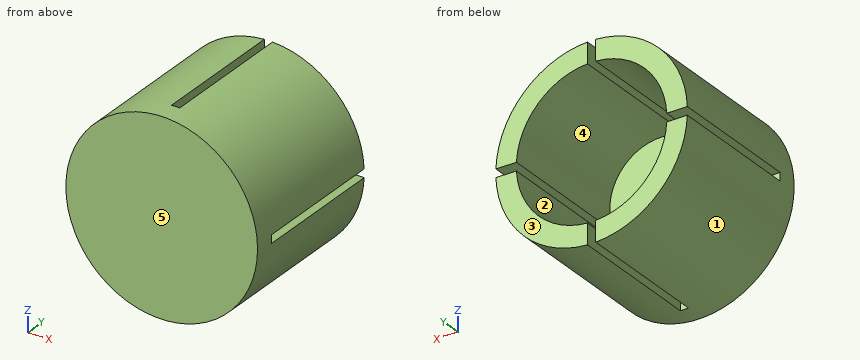
```python
from build123d import *

# Parameters (mm, degrees)
CUT_EXTRUDE1_DEPTH = 20


with BuildPart() as part:
    # Sketch2 → Revolve1 (revolve)
    with BuildSketch(Plane.XY, mode=Mode.PRIVATE) as revolve1_sk:
        Polygon((0, 0), (14, 0), (14, 23), (11, 23), (11, 3), (7.5, 3), (7.5, 8), (0, 8), align=None)
    revolve(revolve1_sk.sketch.rotate(Axis((0, 8, 0), (0, -1, 0)), 180), axis=Axis((0, 8, 0), (0, -1, 0)))

    # Sketch3 → Cut-Extrude1 (cut)
    with BuildSketch(Plane(origin=(0, 23, 0), x_dir=(1, 0, 0), z_dir=(0, 1, 0))):
        with BuildLine():
            ThreePointArc((-0.6, -13.987136948), (-0.300068933, -13.996783868), (0, -14))
            ThreePointArc((0, -14), (0.300068933, -13.996783868), (0.6, -13.987136948))
            Line((0.6, -13.987136948), (0.6, -10.983624174))
            ThreePointArc((0.6, -10.983624174), (0, -11), (-0.6, -10.983624174))
            Line((-0.6, -10.983624174), (-0.6, -13.987136948))
        make_face()
        with BuildLine():
            Line((-0.6, 13.987136948), (-0.6, 10.983624174))
            ThreePointArc((-0.6, 10.983624174), (0, 11), (0.6, 10.983624174))
            Line((0.6, 10.983624174), (0.6, 13.987136948))
            ThreePointArc((0.6, 13.987136948), (0.300068933, 13.996783868), (0, 14))
            ThreePointArc((0, 14), (-0.300068933, 13.996783868), (-0.6, 13.987136948))
        make_face()
        with BuildLine():
            ThreePointArc((-14, 5.1e-08), (-13.996783868, -0.300068907), (-13.987136948, -0.6))
            Line((-13.987136948, -0.6), (-10.983624174, -0.6))
            ThreePointArc((-10.983624174, -0.6), (-11, 0), (-10.983624174, 0.6))
            Line((-10.983624174, 0.6), (-13.987136948, 0.6))
            ThreePointArc((-13.987136948, 0.6), (-13.996783867, 0.300068958), (-14, 5.1e-08))
        make_face()
        with BuildLine():
            Line((10.983624174, -0.6), (13.987136948, -0.6))
            ThreePointArc((13.987136948, -0.6), (13.996783868, -0.300068933), (14, 0))
            ThreePointArc((14, 0), (13.996783868, 0.300068933), (13.987136948, 0.6))
            Line((13.987136948, 0.6), (10.983624174, 0.6))
            ThreePointArc((10.983624174, 0.6), (10.995905281, 0.300111716), (11, 0))
            ThreePointArc((11, 0), (10.995905281, -0.300111716), (10.983624174, -0.6))
        make_face()
    extrude(amount=-CUT_EXTRUDE1_DEPTH, mode=Mode.SUBTRACT)


solid = part.part
```
Work out the finished part from the listing and answer in its coordinate system (mm). Face numbers are marked on the shaded views. A direction names the side the tool comes from. Coordinates: 2 decimals unless noted, no trailing zeros. Loops run counter-clockwise (first coordinate to the right, second up) from the corner with the lowest first, then second, coordinate; pieces in that order, holes last. Notation, with made-up numbers: (-32, 79) -> (-17, 79) arc R38 ccw to (-17, 118) -> close; hole circle Ø5 at (-21, 56). An arc over 180 degrees is marked (long way). Answer as CSV lines item,"result".
Q1. The part is cut by section C-C on z = 0. Write down the section's boundary in (x, y), and give its area (3 significant figures).
Findings:
outline,"(-14, 0) -> (14, 0) -> (14, 3) -> (7.5, 3) -> (7.5, 8) -> (-7.5, 8) -> (-7.5, 3) -> (-14, 3) -> close"
area,"159 mm²"
Q2. Find the intervals of material crossed by probe 1 along Z at (x, y) = (-2.75, 6); probe 2 along Y at (x, z) = (6.75, 4.5); probe 3 along Y at (x, z) = (-0.25, -7), in increasing order.
Findings:
probe 1,"z = -13.73 to -10.65, -6.98 to 6.98, 10.65 to 13.73"
probe 2,"y = 0 to 3"
probe 3,"y = 0 to 8"
Q3. The part is cut by section A-A on y = 4.5. Write down the section's boundary in (x, z), and give its area (3 significant figures).
Findings:
outline,"(-13.99, -0.6) arc R14 ccw to (-0.6, -13.99) -> (-0.6, -10.98) arc R11 cw to (-10.98, -0.6) -> close; (-13.99, 0.6) -> (-10.98, 0.6) arc R11 cw to (-0.6, 10.98) -> (-0.6, 13.99) arc R14 ccw to start; circle Ø15 at (0, 0); (0.6, -13.99) arc R14 ccw to (13.99, -0.6) -> (10.98, -0.6) arc R11 cw to (0.6, -10.98) -> close; (0.6, 10.98) arc R11 cw to (10.98, 0.6) -> (13.99, 0.6) arc R14 ccw to (0.6, 13.99) -> close"
area,"398 mm²"
Q4. A tool of negligible diameter and unlimited length cuts with its end or side. For the marked faces 4 and 5, from which of +Z, -Z, +X, -X, +Y, -Y can it reach the whole face along a straight path? Write none if from no direction.
Findings:
face 4,"+Y"
face 5,"+Z, -Z, +X, -X, -Y"
Q5. For a pull along Z with two mould halves and no side action, classify the marked faces 1, 2 and 3 as +Z half, -Z half, draft (parallel to the pull), parting line (faces both ways), or undercut.
Findings:
face 1,"parting line"
face 2,"undercut"
face 3,"draft"
Q6. The part is cut by section D-D on x = 0. Write down the section's boundary in (y, z), and give its area (3 significant figures).
Findings:
outline,"(0, -14) -> (3, -14) -> (3, -7.5) -> (8, -7.5) -> (8, 7.5) -> (3, 7.5) -> (3, 14) -> (0, 14) -> close"
area,"159 mm²"
Q7. The part is cut by section B-B on y = 9.5. Write down the section's boundary in (x, z), and give its area (3 significant figures).
Findings:
outline,"(-13.99, -0.6) arc R14 ccw to (-0.6, -13.99) -> (-0.6, -10.98) arc R11 cw to (-10.98, -0.6) -> close; (-13.99, 0.6) -> (-10.98, 0.6) arc R11 cw to (-0.6, 10.98) -> (-0.6, 13.99) arc R14 ccw to start; (0.6, -13.99) arc R14 ccw to (13.99, -0.6) -> (10.98, -0.6) arc R11 cw to (0.6, -10.98) -> close; (0.6, 10.98) arc R11 cw to (10.98, 0.6) -> (13.99, 0.6) arc R14 ccw to (0.6, 13.99) -> close"
area,"221 mm²"
Q8. Each of these flat-tipped pins is pushed along its axis until it touches: pin 1 (6 mm diameter, centred on x = 11, y = 3, fed in from -Z); pin 2 (4 mm diameter, centred on x = -4, y = 18, fed in from -Z); pin 3 (12 mm diameter, centred on x = 1, z = -1.5, fed in from +Y); pin 4 (6 mm diameter, centred on x = 6, z = -10.5, fed in from -Y). Where does it stop, or does it pass through?
Findings:
pin 1,"stops at z = -11.49"
pin 2,"stops at z = -13.86"
pin 3,"stops at y = 8"
pin 4,"stops at y = 0"
